Input: part model. Units: mm. Frame: model coordinates. Face numbers are marked on the shaded views. Coordinates: 2 decimals unless noted, no trailing zeros. Loops run counter-clockwise (first coordinate to the right, second up) from the corner with the lowest first, then second, coordinate; pieces in that order, holes last.
(1) Line query: L1, parallel to Y at x = 11.5, z = 1.55; L2, parallel to Y at x = 0, z = 2.1; L3, parallel to X at y = 8.5, z = 2.65. Output: solid intervals per line, ascending.
(2) Section C-C, the plane y = -4. Return loops of the section in (x, z).
(3) Contact query for flat-ended pins moving along their axis: P1, Ø1.5, axis at x = 4, z = 1, coming from the -Y side; P2, Ø1, axis at x = -3.5, z = 2, coming from the -Y side; P3, Ø1.5, axis at x = -13, z = 2.5, coming from the -Y side. Output: stop coordinate, or through.
(4) Section A-A, the plane x = 0. Return loops of the section in (y, z).
(5) Mould query, pull axis Y, two halves, no side actions, for the marked faces 1 and 2. Classes: released by +Y, released by -Y, zero draft, split by the parting line, or undercut.
(6) Section B-B, the plane y = 0. Return loops of the section in (x, z).
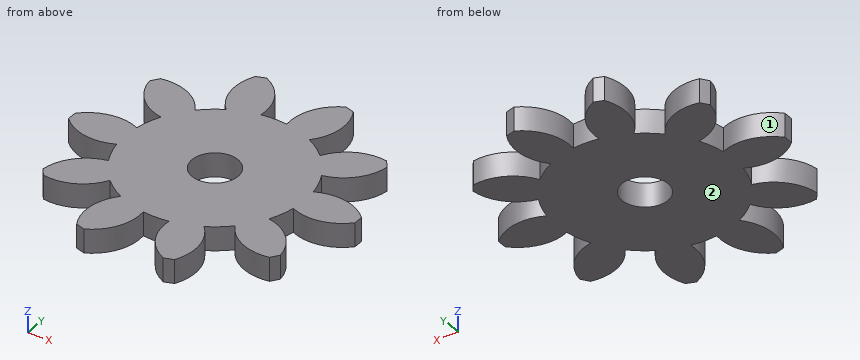
```python
from build123d import *

# Parameters (mm, degrees)
SKETCH1_R           = 18
BOSS_EXTRUDE1_DEPTH = 3
CUT_EXTRUDE2_START  = -3
CUT_EXTRUDE2_DEPTH  = 3
CIRPATTERN1_COUNT   = 10
SKETCH5_R           = 2.9
CUT_EXTRUDE4_DEPTH  = 26.143875003


with BuildPart() as part:
    # Sketch1 → Boss-Extrude1 (new body)
    with BuildSketch(Plane.XY):
        Circle(SKETCH1_R)
    extrude(amount=BOSS_EXTRUDE1_DEPTH)

    # Sketch2 → Cut-Extrude2 (cut)
    with BuildSketch(Plane.XY.offset(3).offset(CUT_EXTRUDE2_START)):
        with BuildLine():
            ThreePointArc((-4.978508794, 17.297816342), (-2.304057127, 14.757459448), (-1.621139762, 11.132583073))
            ThreePointArc((-1.621139762, 11.132583073), (0, 11.25), (1.621139762, 11.132583073))
            ThreePointArc((1.621139762, 11.132583073), (2.304057127, 14.757459448), (4.978508794, 17.297816342))
            ThreePointArc((4.978508794, 17.297816342), (0, 18), (-4.978508794, 17.297816342))
        make_face()
    cut_extrude2 = extrude(amount=CUT_EXTRUDE2_DEPTH, mode=Mode.SUBTRACT)

    # CirPattern1: Cut-Extrude2 ×10 about axis
    cirpattern1_axis = Axis((0, 0, 0), (0, 0, 1))
    for i in range(1, CIRPATTERN1_COUNT):
        add(cut_extrude2.rotate(cirpattern1_axis, i * 360 / CIRPATTERN1_COUNT), mode=Mode.SUBTRACT)

    # Sketch5 → Cut-Extrude4 (cut, through all)
    with BuildSketch(Plane.XY.offset(3)):
        Circle(SKETCH5_R)
    extrude(amount=-CUT_EXTRUDE4_DEPTH, mode=Mode.SUBTRACT)


solid = part.part
```
Report:
1. L1: y = -10.94 to -5.44, -2.07 to 2.07, 5.44 to 10.94
1. L2: y = -11.25 to -2.9, 2.9 to 11.25
1. L3: x = -14.48 to -8.13, -7.37 to 7.37, 8.13 to 14.48
2. outline: (-10.51, 0) - (10.51, 0) - (10.51, 3) - (-10.51, 3) - close
3. P1: stops at y = -17.18
3. P2: stops at y = -16.71
3. P3: stops at y = -11.17
4. outline: (-11.25, 0) - (-2.9, 0) - (-2.9, 3) - (-11.25, 3) - close; (2.9, 0) - (11.25, 0) - (11.25, 3) - (2.9, 3) - close
5. face 1: undercut
5. face 2: zero draft
6. outline: (-18, 0) - (-2.9, 0) - (-2.9, 3) - (-18, 3) - close; (2.9, 0) - (18, 0) - (18, 3) - (2.9, 3) - close
